from build123d import *

# Parameters (mm, degrees)
F1_R     = 19.05
F2_DEPTH = 101.6
F0_R     = 38.1
F3_DEPTH = 50.8


with BuildPart() as f2:
    # F1 (on Front) → F2 (new body, symmetric)
    with BuildSketch(Plane.XZ):
        Circle(F1_R)
    extrude(amount=F2_DEPTH, both=True)

    # F0 (on Front) → F3 (join, symmetric)
    with BuildSketch(Plane.XZ):
        Circle(F0_R)
    extrude(amount=F3_DEPTH, both=True)


solid = f2.part
Verification items for the finished model (mm, model axes). A direction names the side the tool comes from. Coordinates: 2 decimals unless noted, no trailing zeros. Order: outer loops, then holes, each group sorted by start corner. A loop starts at its lowest first (then second) coordinate and runs counter-clockwise, first axis right, second up. Notation, with made-up numbers: M -14,-1.5 L 15,-1.5 A22 cw 15,15.5 Z; hole C 21.25,-33.75 d3. An arc over 180 degrees is marked long. One line per item, written item: value. Start each with the question number.
Item 1: Scan lines: probe 1 along Y at (x, z) = (12, -26.5); probe 2 along X at (y, z) = (-12.5, 33); probe 3 along X at (y, z) = (42, -25). Record each from-to range of solid material in increasing order.
Item 2: Sectioned sample at B-B (z = 0). Enter the section's corners in (x, y).
Item 3: Gauge pin test, flat ends, axial feed: pin 1 (5 mm diameter, centred on x = -27.5, z = -4, fed in from -Y); pin 2 (6 mm diameter, centred on y = 40.5, z = -24, fed in from -X); pin 3 (5 mm diameter, centred on y = -69, z = -17, fed in from +X); pin 4 (2 mm diameter, centred on x = 21, y = 55.5, fed in from +Z). Record the tip position at first contact, or that the pin passes through.
Item 4: Sectioned sample at C-C (y = -85). Enter the section's corners in (x, z).
Item 5: Sectioned sample at A-A (x = 0). Enter the section's corners in (y, z), then the cut area to 3 significant figures.
Item 6: Access from +Z, -Z, +X, -X, +Y, -Y to the whole of each face (thin tool, end or side, straight path). Record for faces 1 (the flat face through (0, -101.6, 0)), 2 (the cylindrical face through (-15.12, -76.56, -11.59)), 3 (the cylindrical face through (-15.12, 75.84, -11.59)).
Item 7: Sectioned sample at D-D (y = 29). Enter the section's corners in (x, z).
Conclusion:
1. probe 1: y = -50.8 to 50.8
1. probe 2: x = -19.04 to 19.04
1. probe 3: x = -28.75 to 28.75
2. outline: M -38.1,-50.8 L -19.05,-50.8 L -19.05,-101.6 L 19.05,-101.6 L 19.05,-50.8 L 38.1,-50.8 L 38.1,50.8 L 19.05,50.8 L 19.05,101.6 L -19.05,101.6 L -19.05,50.8 L -38.1,50.8 Z
3. pin 1: stops at y = -50.8
3. pin 2: stops at x = -31.79
3. pin 3: stops at x = 12.36
3. pin 4: passes through
4. outline: C 0,0 d38.1
5. outline: M -101.6,-19.05 L -50.8,-19.05 L -50.8,-38.1 L 50.8,-38.1 L 50.8,-19.05 L 101.6,-19.05 L 101.6,19.05 L 50.8,19.05 L 50.8,38.1 L -50.8,38.1 L -50.8,19.05 L -101.6,19.05 Z
5. area: 11,600 mm^2
6. face 1: +Z, -Z, +X, -X, -Y
6. face 2: -Y
6. face 3: +Y
7. outline: C 0,0 d76.2
